Check sheet for the modelled part. Datum: model origin and axes. Units: mm. A direction names the side the tool comes from. Round coordinates to 2 decimals unless told otherwise and drop trailing zeros. Loops run counter-clockwise (first coordinate to the right, second up) from the corner with the lowest first, then second, coordinate; pieces in that order, holes last. Notation, with made-up numbers: (27, 38) - (37, 38) arc R11 cw to (37, 43) - close; hole circle Ø6 at (6.5, -9). An arc over 180 degrees is marked (long way). Put each result on its own line as item: value.
```python
from build123d import *

# Parameters (mm, degrees)
SKETCH_1_W          = 4
SKETCH_1_H          = 3.5
SKETCH_2_R          = 2
EXTRUDE_1_DEPTH     = 45
CUT_EXTRUDE_1_DEPTH = 2
CHAMFER_1_SIZE      = 0.6062
CHAMFER_1_SIZE2     = 0.35
FILLET_1_R          = 0.2


with BuildPart() as part:
    # 草图1 → 旋转1 (revolve)
    with BuildSketch(Plane.XY):
        with Locations((2, 1.75)):
            Rectangle(SKETCH_1_W, SKETCH_1_H)
    revolve(axis=Axis((0, 0, 0), (1, 0, 0)))

    # 草图2 → 凸台-拉伸1 (add)
    with BuildSketch(Plane(origin=(4, 0, 0), x_dir=(0, 0, -1), z_dir=(1, 0, 0))):
        Circle(SKETCH_2_R)
    extrude(amount=EXTRUDE_1_DEPTH)

    # 草图3 → 切除-拉伸1 (cut)
    with BuildSketch(Plane.ZY):
        Polygon((0, 1.72), (-1.489563695, 0.86), (-1.489563695, -0.86), (0, -1.72), (1.489563695, -0.86), (1.489563695, 0.86), align=None)
    extrude(amount=-CUT_EXTRUDE_1_DEPTH, mode=Mode.SUBTRACT)

    # 倒角1
    chamfer_1_edges = [part.edges().sort_by_distance(p)[0] for p in [
        (49, 0, 2),
    ]]
    chamfer_1_side = [part.faces().sort_by_distance(p)[0] for p in [
        (49, 0, 0),
    ]]
    chamfer(chamfer_1_edges, length=CHAMFER_1_SIZE, length2=CHAMFER_1_SIZE2, reference=chamfer_1_side[0])

    # 圆角1
    fillet_1_edges = [part.edges().sort_by_distance(p)[0] for p in [
        (0, -3.5, 0),
        (4, 0, 2),
    ]]
    fillet(fillet_1_edges, radius=FILLET_1_R)


solid = part.part
```
Item 1: Go/stop test with flat-tipped pins: pin 1 (4 mm diameter, centred on x = 11.5, y = 0, fed in from +Z); pin 2 (4 mm diameter, centred on x = 8.5, z = -2, fed in from -Y); pin 3 (1.5 mm diameter, centred on x = 37.5, z = 1.5, fed in from -Y). Record where each tip stops, or that it passes through.
Filled sheet:
pin 1: z = 2
pin 2: y = -2
pin 3: y = -1.85
Item 2: Section check A-A on y = 0. Enter the section's corners in (x, z).
Filled sheet:
outline: (0, -3.3) arc R0.2 ccw to (0.2, -3.5) - (4, -3.5) - (4, -2.2) arc R0.2 cw to (4.2, -2) - (48.65, -2) - (49, -1.39) - (49, 1.39) - (48.65, 2) - (4.2, 2) arc R0.2 cw to (4, 2.2) - (4, 3.5) - (0.2, 3.5) arc R0.2 ccw to (0, 3.3) - (0, 1.49) - (2, 1.49) - (2, -1.49) - (0, -1.49) - close
Item 3: Release check for a two-part mould opening along Y. For faces 3 (the flat face through (0.99, 1.28, 0.76)), 4 (the flat face through (4, 2, -2)), 5 (the cylindrical face through (26, -2, 0)) record: +Y half, -Y half, draft (parallel to the pull), parting line (faces both ways), or undercut.
Filled sheet:
face 3: undercut
face 4: draft
face 5: parting line
Item 4: Tool access check on faces 1 (the flat face through (0, 0, 2)), 2 (the flat face through (0.99, -1.28, -0.76)). Record the directions out of +Z, -Z, +X, -X, +Y, -Y that give a thin tool (end or side, any length) a straight path to the whole face; none if there is none.
Filled sheet:
face 1: +Z, -Z, -X, +Y, -Y
face 2: -X
Item 5: Thickness scan on line 1 (X direction, y = 0.75, z = 2.75); line 2 (X direction, y = 0.25, z = 0.25); line 3 (Y direction, x = 5, z = 0). Record the ranges inside material, lowest first. Write a range as from..to.
Filled sheet:
line 1: 0..4
line 2: 2..49
line 3: -2..2
Item 6: Section check B-B on x = 16.5. Enter the section's corners in (y, z), then the cut area to 3 significant figures.
Filled sheet:
outline: circle Ø4 at (0, 0)
area: 12.6 mm²
